Design review of the part built by this model. Coordinates are the model's own, in mm. A direction names the side the tool comes from. Give positions to 0.01 mm unless a question says otherwise; leave off trailing zeros. Loops run counter-clockwise (first coordinate to the right, second up) from the corner with the lowest first, then second, coordinate; pieces in that order, holes last.
from build123d import *

# Parameters (mm, degrees)
BOSS_EXTRUDE1_DEPTH = 6.604
CUT_EXTRUDE1_DEPTH  = 7.604
FILLET1_R           = 12.7
CUT_EXTRUDE2_DEPTH  = 7.604
SKETCH5_W           = 6.35
SKETCH5_H           = 6.35
BOSS_EXTRUDE2_DEPTH = 6.604
SKETCH6_W           = 10.16
SKETCH6_H           = 22.225
CUT_EXTRUDE5_DEPTH  = 7.604
FILLET2_R           = 2.54


with BuildPart() as part:
    # Sketch1 → Boss-Extrude1 (new body)
    with BuildSketch(Plane(origin=(0, 0, 0), x_dir=(1, 0, 0), z_dir=(0, 1, 0))):
        Polygon((44.45, -152.4), (76.2, -152.4), (76.2, 0), (-76.2, 0), (-76.2, -152.4), (-44.45, -152.4), (-44.45, -31.75), (44.45, -31.75), align=None)
    extrude(amount=BOSS_EXTRUDE1_DEPTH)

    # Sketch2 → Cut-Extrude1 (cut, through all)
    with BuildSketch(Plane(origin=(0, 6.604, 0), x_dir=(1, 0, 0), z_dir=(0, 1, 0))):
        with BuildLine():
            Line((-56.8325, -25.4), (-56.8325, -127))
            ThreePointArc((-56.8325, -127), (-60.325, -130.4925), (-63.8175, -127))
            Line((-63.8175, -127), (-63.8175, -25.4))
            ThreePointArc((-63.8175, -25.4), (-60.325, -21.9075), (-56.8325, -25.4))
        make_face()
        with BuildLine():
            Line((56.8325, -25.4), (56.8325, -127))
            ThreePointArc((56.8325, -127), (60.325, -130.4925), (63.8175, -127))
            Line((63.8175, -127), (63.8175, -25.4))
            ThreePointArc((63.8175, -25.4), (60.325, -21.9075), (56.8325, -25.4))
        make_face()
    extrude(amount=-CUT_EXTRUDE1_DEPTH, mode=Mode.SUBTRACT)

    # Fillet1
    fillet1_edges = [part.edges().sort_by_distance(p)[0] for p in [
        (76.2, 3.302, 152.4),
        (44.45, 3.302, 152.4),
        (44.45, 3.302, 31.75),
        (-44.45, 3.302, 31.75),
        (-44.45, 3.302, 152.4),
        (-76.2, 3.302, 152.4),
    ]]
    fillet(fillet1_edges, radius=FILLET1_R)

    # Sketch4 → Cut-Extrude2 (cut, through all)
    with BuildSketch(Plane(origin=(0, 6.604, 0), x_dir=(1, 0, 0), z_dir=(0, 1, 0))):
        Polygon((-40.1828, 0), (-40.1828, -6.35), (-42.4688, -6.35), (-42.4688, -12.2936), (-40.1828, -12.2936), (-40.1828, -13.97), (-36.0172, -13.97), (-36.0172, -12.2936), (-33.7312, -12.2936), (-33.7312, -6.35), (-36.0172, -6.35), (-36.0172, 0), align=None)
        Polygon((36.0172, 0), (36.0172, -6.35), (33.7312, -6.35), (33.7312, -12.2936), (36.0172, -12.2936), (36.0172, -13.97), (40.1828, -13.97), (40.1828, -12.2936), (42.4688, -12.2936), (42.4688, -6.35), (40.1828, -6.35), (40.1828, 0), align=None)
    extrude(amount=-CUT_EXTRUDE2_DEPTH, mode=Mode.SUBTRACT)

    # Sketch5 → Boss-Extrude2 (add)
    with BuildSketch(Plane(origin=(0, 6.604, 0), x_dir=(1, 0, 0), z_dir=(0, 1, 0))):
        with Locations((-47.625, 3.175)):
            Rectangle(SKETCH5_W, SKETCH5_H)
        with Locations((-28.575, 3.175)):
            Rectangle(SKETCH5_W, SKETCH5_H)
        with Locations((47.625, 3.175)):
            Rectangle(SKETCH5_W, SKETCH5_H)
        with Locations((28.575, 3.175)):
            Rectangle(SKETCH5_W, SKETCH5_H)
    extrude(amount=-BOSS_EXTRUDE2_DEPTH)

    # Sketch6 → Cut-Extrude5 (cut, through all)
    with BuildSketch(Plane(origin=(0, 6.604, 0), x_dir=(1, 0, 0), z_dir=(0, 1, 0))):
        with Locations((-19.05, -20.6375)):
            Rectangle(SKETCH6_W, SKETCH6_H)
        with Locations((19.05, -20.6375)):
            Rectangle(SKETCH6_W, SKETCH6_H)
    extrude(amount=-CUT_EXTRUDE5_DEPTH, mode=Mode.SUBTRACT)

    # Fillet2
    fillet2_edges = [part.edges().sort_by_distance(p)[0] for p in [
        (-24.13, 3.302, 31.75),
        (-24.13, 3.302, 9.525),
        (-13.97, 3.302, 9.525),
        (-13.97, 3.302, 31.75),
        (13.97, 3.302, 31.75),
        (13.97, 3.302, 9.525),
        (24.13, 3.302, 9.525),
        (24.13, 3.302, 31.75),
    ]]
    fillet(fillet2_edges, radius=FILLET2_R)


solid = part.part
Q1. Tool access review of faces 5 (the face through (13.97, 3, 21)), 6 (the face through (-63, 3, 0)), 7 (the face through (42.469, 3, 9)): name each direction out of +Z, -Z, +X, -X, +Y, -Y from which nothing blocks a thin tool from reaching the whole face with its end or side.
Results:
face 5: +Z, +Y, -Y
face 6: -Z, -X, +Y, -Y
face 7: +Y, -Y
Q2. Take a section at D-D (z = 34.5). Give the boundary of the cut face in (x, y), plus the area to 3 significant figures.
Results:
outline: (-76.2, 0) - (-63.82, 0) - (-63.82, 6.6) - (-76.2, 6.6) - close; (-56.83, 0) - (-39.64, 0) - (-39.64, 6.6) - (-56.83, 6.6) - close; (39.64, 0) - (56.83, 0) - (56.83, 6.6) - (39.64, 6.6) - close; (63.82, 0) - (76.2, 0) - (76.2, 6.6) - (63.82, 6.6) - close
area: 391 mm2
Q3. Take a section at C-C (x = -8). Give the boundary of the cut face in (y, z), plus the area to 3 significant figures.
Results:
outline: (0, 0) - (6.6, 0) - (6.6, 31.75) - (0, 31.75) - close
area: 210 mm2
Q4. Insertion check: pin 1 (1.5 mm diameter, centred on x = -19.5, y = 3.5, fed in from +Z) (3 decimals); pin 2 (3.5 mm diameter, centred on x = 42.5, y = 2.5, fed in from -Z); pin 3 (2.5 mm diameter, centred on x = 42, y = 3, fed in from +Z). Each pin has a flat end and moves straight along its axis. Give the tip position at first contact, or say it passes through.
Results:
pin 1: stops at z = 9.525
pin 2: stops at z = 0
pin 3: stops at z = 39.06
Q5. Take a section at A-A (z = 124). Give the boundary of the cut face in (x, y).
Results:
outline: (-76.2, 0) - (-63.82, 0) - (-63.82, 6.6) - (-76.2, 6.6) - close; (-56.83, 0) - (-44.45, 0) - (-44.45, 6.6) - (-56.83, 6.6) - close; (44.45, 0) - (56.83, 0) - (56.83, 6.6) - (44.45, 6.6) - close; (63.82, 0) - (76.2, 0) - (76.2, 6.6) - (63.82, 6.6) - close
Q6. Wall thickness on line 1 (X direction, y = 2.5, z = 55); line 2 (X direction, y = 6, z = 14.5); line 3 (X direction, y = 2.25, z = 35.5): over which ranges is each line inside the solid? List them lowest first.
Results:
line 1: x = -76.2 to -63.82, -56.83 to -44.45, 44.45 to 56.83, 63.82 to 76.2
line 2: x = -76.2 to -24.13, -13.97 to 13.97, 24.13 to 76.2
line 3: x = -76.2 to -63.82, -56.83 to -40.76, 40.76 to 56.83, 63.82 to 76.2
Q7. Take a section at B-B (y = 4). Give the number of separate pieces and of enclosed holes in the cut face, plus the area to 3 significant figures.
Results:
separate pieces: 1
enclosed holes: 2
area: 10,500 mm2
Q8. Draft analysis for pull direction X (two halves, no side actions). For faces 1 (the face through (76.2, 3, 71)), 2 (the face through (19, 3, 9.525)), 3 (the face through (-50.8, 3, -3)), 4 (the face through (44.45, 3, 91)), state which applies: pulls with the +X half, pulls with the -X half, needs draft (parallel to the pull), parting line crosses it, or undercut.
Results:
face 1: pulls with the +X half
face 2: undercut
face 3: pulls with the -X half
face 4: undercut
